Geometry: final body of the model. Coordinates: model frame, mm. Face numbers are marked on the shaded views. A direction names the side the tool comes from. Give positions to 0.01 mm unless a question says otherwise; leave off trailing zeros. Loops run counter-clockwise (first coordinate to the right, second up) from the corner with the lowest first, then second, coordinate; pieces in that order, holes last. Notation, with made-up numbers: (76.25, 85.25) - (131.25, 85.25) arc R20 ccw to (131.25, 109.25) - close; hole circle Ø7 at (75.25, 12.5). An arc over 180 degrees is marked (long way). Use one line per item in the form item = value.
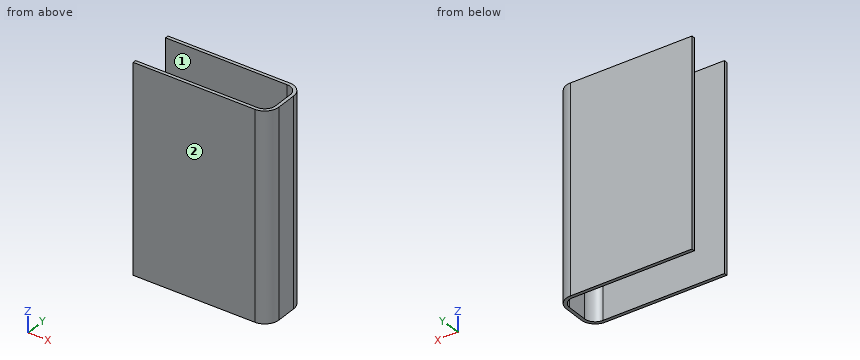
```python
from build123d import *

# Parameters (mm, degrees)
SKETCH3_W                       = 304.8
SKETCH3_H                       = 0.79375
BOSS_EXTRUDE1_DEPTH             = 152.4
BOSS_EXTRUDE1_DEPTH_BACK        = 152.4
SKETCH4_OUTSIDE_W               = 393.01
SKETCH4_OUTSIDE_H               = 393.01
SKETCH4_OUTSIDE_W_2             = 28.9306
SKETCH4_OUTSIDE_H_2             = 48.9966
CUT_EXTRUDE1_DEPTH              = 1.396875
CUT_EXTRUDE1_DEPTH_BACK         = 1.396875
EXTRUDE_THIN1_REACH             = 26.498
EXTRUDE_THIN1_DIRECTION_2_REACH = 26.498


with BuildPart() as part:
    # Sketch3 → Boss-Extrude1 (new body, two sides)
    with BuildSketch(Plane.XY) as boss_extrude1_sk:
        Rectangle(SKETCH3_W, SKETCH3_H)
    extrude(amount=BOSS_EXTRUDE1_DEPTH)
    extrude(boss_extrude1_sk.sketch, amount=-BOSS_EXTRUDE1_DEPTH_BACK)

    # Sketch4 outside → Cut-Extrude1 (cut, two sides)
    with BuildSketch(Plane(origin=(0, 0, 0), x_dir=(1, 0, 0), z_dir=(0, 1, 0))) as cut_extrude1_sk:
        Rectangle(SKETCH4_OUTSIDE_W, SKETCH4_OUTSIDE_H)
        with Locations((-137.9347, -127.9017)):
            Rectangle(SKETCH4_OUTSIDE_W_2, SKETCH4_OUTSIDE_H_2, mode=Mode.SUBTRACT)
    extrude(amount=CUT_EXTRUDE1_DEPTH, mode=Mode.SUBTRACT)
    extrude(cut_extrude1_sk.sketch, amount=-CUT_EXTRUDE1_DEPTH_BACK, mode=Mode.SUBTRACT)

    # Extrude-Thin1: up to this face of the body (flat: up to its plane)
    extrude_thin1_end = Plane(part.part.faces().sort_by_distance((-137.9347, 0, 103.4034))[0])
    # Sketch5 → Extrude-Thin1 (add, up to the picked face)
    with BuildSketch(Plane.XY.offset(127.9017), mode=Mode.PRIVATE) as extrude_thin1_sk1:
        with BuildLine():
            Line((-152.4, -10.404475), (-123.4694, -10.404475))
            ThreePointArc((-123.4694, -10.404475), (-121.673348776, -9.660526224), (-120.9294, -7.864475))
            Line((-120.9294, -7.864475), (-120.9294, -2.936875))
            ThreePointArc((-120.9294, -2.936875), (-121.673348776, -1.140823776), (-123.4694, -0.396875))
            Line((-123.4694, -0.396875), (-123.4694, 0.396875))
            ThreePointArc((-123.4694, 0.396875), (-121.112082768, -0.579557768), (-120.13565, -2.936875))
            Line((-120.13565, -2.936875), (-120.13565, -7.864475))
            ThreePointArc((-120.13565, -7.864475), (-121.112082768, -10.221792232), (-123.4694, -11.198225))
            Line((-123.4694, -11.198225), (-152.4, -11.198225))
            Line((-152.4, -11.198225), (-152.4, -10.404475))
        make_face()
    extrude_thin1_tool1 = split(extrude(extrude_thin1_sk1.sketch, amount=-EXTRUDE_THIN1_REACH, mode=Mode.PRIVATE), bisect_by=extrude_thin1_end, keep=Keep.BOTH, mode=Mode.PRIVATE)
    add(extrude_thin1_tool1.solids().sort_by_distance((-137.9347, -10.855379, 127.9017))[0])

    # Extrude-Thin1 direction 2: up to this face of the body (flat: up to its plane)
    extrude_thin1_direction_2_end = Plane(part.part.faces().sort_by_distance((-137.9347, 0, 152.4))[0])
    # Sketch5 → Extrude-Thin1 direction 2 (add, up to the picked face)
    with BuildSketch(Plane.XY.offset(127.9017), mode=Mode.PRIVATE) as extrude_thin1_direction_2_sk1:
        with BuildLine():
            Line((-152.4, -10.404475), (-123.4694, -10.404475))
            ThreePointArc((-123.4694, -10.404475), (-121.673348776, -9.660526224), (-120.9294, -7.864475))
            Line((-120.9294, -7.864475), (-120.9294, -2.936875))
            ThreePointArc((-120.9294, -2.936875), (-121.673348776, -1.140823776), (-123.4694, -0.396875))
            Line((-123.4694, -0.396875), (-123.4694, 0.396875))
            ThreePointArc((-123.4694, 0.396875), (-121.112082768, -0.579557768), (-120.13565, -2.936875))
            Line((-120.13565, -2.936875), (-120.13565, -7.864475))
            ThreePointArc((-120.13565, -7.864475), (-121.112082768, -10.221792232), (-123.4694, -11.198225))
            Line((-123.4694, -11.198225), (-152.4, -11.198225))
            Line((-152.4, -11.198225), (-152.4, -10.404475))
        make_face()
    extrude_thin1_direction_2_tool1 = split(extrude(extrude_thin1_direction_2_sk1.sketch, amount=EXTRUDE_THIN1_DIRECTION_2_REACH, mode=Mode.PRIVATE), bisect_by=extrude_thin1_direction_2_end, keep=Keep.BOTH, mode=Mode.PRIVATE)
    add(extrude_thin1_direction_2_tool1.solids().sort_by_distance((-137.9347, -10.855379, 127.9017))[0])


solid = part.part
```
(1) Access query for the marked faces 1 and 2. Directions: +Z, -Z, +X, -X, +Y, -Y. A direction counts if a zero-diameter tool reaches every point of the face in a straight line with its end or side. Return the directions, or none.
Solution:
face_1 = +Z, -Z, -X
face_2 = +Z, -Z, +X, -X, -Y
(2) Pin query (flat end, axial travel): P1, Ø1.5, axis at y = -9, z = 113.5, coming from the -X side; P2, Ø1.5, axis at y = -6, z = 116, coming from the -X side. Return the tip coordinate at first contact, or that it passes through.
Solution:
P1 = -121.77
P2 = -120.93
(3) Cut plane C-C (y = -4.25). Return the cut outline in (x, z), plus the area to 3 significant figures.
Solution:
outline = (-120.93, 103.4) - (-120.14, 103.4) - (-120.14, 152.4) - (-120.93, 152.4) - close
area = 38.9 mm2
(4) Cut plane B-B (z = 109). Return the cut outline in (x, y).
Solution:
outline = (-152.4, -11.2) - (-123.47, -11.2) arc R3.33 ccw to (-120.14, -7.86) - (-120.14, -2.94) arc R3.33 ccw to (-123.47, 0.4) - (-152.4, 0.4) - (-152.4, -0.4) - (-123.47, -0.4) arc R2.54 cw to (-120.93, -2.94) - (-120.93, -7.86) arc R2.54 cw to (-123.47, -10.4) - (-152.4, -10.4) - close
(5) Cut plane A-A (x = -139). Return the cut outline in (y, z), plus the area to 3 significant figures.
Solution:
outline = (-11.2, 103.4) - (-10.4, 103.4) - (-10.4, 152.4) - (-11.2, 152.4) - close; (-0.4, 103.4) - (0.4, 103.4) - (0.4, 152.4) - (-0.4, 152.4) - close
area = 77.8 mm2
(6) Material intervals for L1, parallel to Y at x = -134, z = 126; L2, parallel to X at y = -3.75, z = 148.5; L3, parallel to Y at x = -122, z = 135, sorted ascending. Write a range as from..to.
Solution:
L1 = -11.2..-10.4, -0.4..0.4
L2 = -120.93..-120.14
L3 = -10.86..-9.94, -0.87..0.06
(7) Cut plane D-D (y = -8.5). Return the cut outline in (x, z).
Solution:
outline = (-121.01, 103.4) - (-120.2, 103.4) - (-120.2, 152.4) - (-121.01, 152.4) - close
